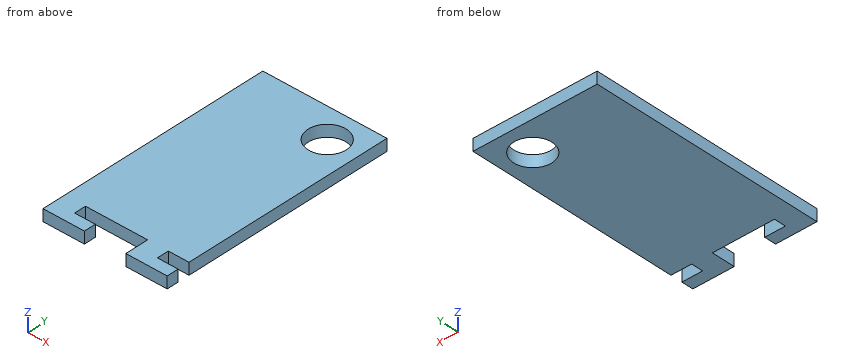
```python
from build123d import *

# Parameters (mm, degrees)
SKETCH1_W           = 50.8
SKETCH1_H           = 96.655493252
BOSS_EXTRUDE1_DEPTH = 4.800000052
SKETCH3_R           = 7.8277466
CUT_EXTRUDE2_DEPTH  = 110.297595473
SKETCH4_W           = 8.466666667
SKETCH4_H           = 4.800000052
SKETCH4_W_2         = 8.466666666
CUT_EXTRUDE4_DEPTH  = 110.297595473
SKETCH5_W           = 16.933333334
SKETCH5_H           = 9.600000104
CUT_EXTRUDE5_DEPTH  = 110.297595473


with BuildPart() as part:
    # Sketch1 → Boss-Extrude1 (new body)
    with BuildSketch(Plane.XY):
        with Locations((25.4, 48.327746626)):
            Rectangle(SKETCH1_W, SKETCH1_H)
    extrude(amount=BOSS_EXTRUDE1_DEPTH)

    # Sketch3 → Cut-Extrude2 (cut, through all)
    with BuildSketch(Plane(origin=(0, 0, 0), x_dir=(-1, 0, 0), z_dir=(0, 0, -1))):
        with Locations((-38.1, 84.0277466)):
            Circle(SKETCH3_R)
    extrude(amount=-CUT_EXTRUDE2_DEPTH, mode=Mode.SUBTRACT)

    # Sketch4 → Cut-Extrude4 (cut, through all)
    with BuildSketch(Plane(origin=(0, 0, 0), x_dir=(-1, 0, 0), z_dir=(0, 0, -1))):
        with Locations((-46.566666667, 7.200000078)):
            Rectangle(SKETCH4_W, SKETCH4_H)
        with Locations((-12.7, 7.200000078)):
            Rectangle(SKETCH4_W_2, SKETCH4_H)
    extrude(amount=-CUT_EXTRUDE4_DEPTH, mode=Mode.SUBTRACT)

    # Sketch5 → Cut-Extrude5 (cut, through all)
    with BuildSketch(Plane(origin=(0, 0, 0), x_dir=(-1, 0, 0), z_dir=(0, 0, -1))):
        with Locations((-25.4, 4.800000052)):
            Rectangle(SKETCH5_W, SKETCH5_H)
    extrude(amount=-CUT_EXTRUDE5_DEPTH, mode=Mode.SUBTRACT)


solid = part.part
```
The listing builds one solid part. Answer for the finished solid, in the listing's coordinates (mm). Round coordinates to 2 decimals unless told otherwise and drop trailing zeros. Loops run counter-clockwise (first coordinate to the right, second up) from the corner with the lowest first, then second, coordinate; pieces in that order, holes last.
Q1. Section D-D, the plane x = 26.5 is taken. Determine the outline of the cut face in (y, z).
Q2. Given pin 1 Ø2.5 at (y, z) = (7, 1.5) entering from -X; pin 2 Ø2.5 at (y, z) = (7.5, 2) entering from +X; pin 3 Ø1.4 at (x, z) = (25.5, 1.5) entering from -Y, each flat-ended and moving along its own axis, determine where each tip first touches the part or whether it passes through.
Q3. Find the intervals of material crossed by line 1 (Y direction, x = 38.1, z = 2.5); line 2 (Y direction, x = 16, z = 0.2); line 3 (X direction, y = 7.5, z = 3.4), in increasing order.
Q4. Section B-B, the plane x = 15 is taken. Determine the outline of the cut face in (y, z).
Q5. Section C-C, the plane z = 3 is taken. Determine the outline of the cut face in (x, y).
Q6. Section A-A, the plane x = 38.1 is taken. Determine the outline of the cut face in (y, z), then the cut area to 3 significant figures.
Completed:
1. outline: (9.6, 0) - (96.66, 0) - (96.66, 4.8) - (9.6, 4.8) - close
2. pin 1: stops at x = 0
2. pin 2: stops at x = 42.33
2. pin 3: stops at y = 9.6
3. line 1: y = 0 to 76.2, 91.86 to 96.66
3. line 2: y = 0 to 4.8, 9.6 to 96.66
3. line 3: x = 0 to 8.47, 33.87 to 42.33
4. outline: (0, 0) - (4.8, 0) - (4.8, 4.8) - (0, 4.8) - close; (9.6, 0) - (96.66, 0) - (96.66, 4.8) - (9.6, 4.8) - close
5. outline: (0, 0) - (16.93, 0) - (16.93, 4.8) - (8.47, 4.8) - (8.47, 9.6) - (33.87, 9.6) - (33.87, 0) - (50.8, 0) - (50.8, 4.8) - (42.33, 4.8) - (42.33, 9.6) - (50.8, 9.6) - (50.8, 96.66) - (0, 96.66) - close; hole circle Ø15.66 at (38.1, 84.03)
6. outline: (0, 0) - (76.2, 0) - (76.2, 4.8) - (0, 4.8) - close; (91.86, 0) - (96.66, 0) - (96.66, 4.8) - (91.86, 4.8) - close
6. area: 389 mm2
